from build123d import *

# Parameters (mm, degrees)
SKETCH1_R           = 1.75
SKETCH1_R_2         = 11.5
BOSS_EXTRUDE1_DEPTH = 3.55


with BuildPart() as part:
    # Sketch1 → Boss-Extrude1 (new, symmetric)
    with BuildSketch(Plane.XY):
        Polygon((21.15, -17.614466094), (21.15, 17.614466094), (17.614466094, 21.15), (-17.614466094, 21.15), (-21.15, 17.614466094), (-21.15, -17.614466094), (-17.614466094, -21.15), (17.614466094, -21.15), align=None)
        with Locations((-15.5, 15.5)):
            Circle(SKETCH1_R, mode=Mode.SUBTRACT)
        with Locations((15.5, 15.5)):
            Circle(SKETCH1_R, mode=Mode.SUBTRACT)
        with Locations((15.5, -15.5)):
            Circle(SKETCH1_R, mode=Mode.SUBTRACT)
        with Locations((-15.5, -15.5)):
            Circle(SKETCH1_R, mode=Mode.SUBTRACT)
        Circle(SKETCH1_R_2, mode=Mode.SUBTRACT)
    extrude(amount=BOSS_EXTRUDE1_DEPTH, both=True)


solid = part.part
Design review of the part built by this model. Coordinates are the model's own, in mm. Round coordinates to 2 decimals unless told otherwise and drop trailing zeros. Write each loop counter-clockwise with the first axis right and the second up, starting at its lowest first coordinate (ties: lowest second). Pieces come first, ordered by that corner, then holes. Notation, with made-up numbers: (55.25, 57) - (66.25, 57) arc R7 cw to (66.25, 62) - close; hole circle Ø1 at (-22, -18). An arc over 180 degrees is marked (long way). Use a Markdown table: item, result. Add a question column.
1. We need section C-C (z = -0.5). State the section outline as (x, y) points.
2. Wall thickness on probe 1 along Y at (x, z) = (-15.5, 0); probe 2 along Y at (x, z) = (0, 0.75); probe 3 along Y at (x, z) = (-14, -3): over which ranges is each line inside the solid? List them lowest first.
3. Mouldability with a two-part tool opening along Y and no side actions: class faces 1 (the face through (-1.5, 11.4, 0)), 2 (the face through (-14.6, -14, 0)), 3 (the face through (-21.15, 0, 0)), 4 (the face through (-19.407, -19.357, 0.05)) as +Y half, -Y half, draft (parallel to the pull), parting line (faces both ways), or undercut.
4. We need section B-B (x = 15.5). State the section outline as (y, z) points, then the cut area to 3 significant figures.
5. We need section A-A (y = 0). State the section outline as (x, z) points, then the cut area to 3 significant figures.
Output:
| question | item | result |
|---|---|---|
| 1 | outline | (-21.15, -17.61) - (-17.61, -21.15) - (17.61, -21.15) - (21.15, -17.61) - (21.15, 17.61) - (17.61, 21.15) - (-17.61, 21.15) - (-21.15, 17.61) - close; hole circle Ø3.5 at (-15.5, -15.5); hole circle Ø3.5 at (-15.5, 15.5); hole circle Ø23 at (0, 0); hole circle Ø3.5 at (15.5, -15.5); hole circle Ø3.5 at (15.5, 15.5) |
| 2 | probe 1 | y = -21.15 to -17.25, -13.75 to 13.75, 17.25 to 21.15 |
| 2 | probe 2 | y = -21.15 to -11.5, 11.5 to 21.15 |
| 2 | probe 3 | y = -21.15 to -16.4, -14.6 to 14.6, 16.4 to 21.15 |
| 3 | face 1 | undercut |
| 3 | face 2 | undercut |
| 3 | face 3 | draft |
| 3 | face 4 | -Y half |
| 4 | outline | (-21.15, -3.55) - (-17.25, -3.55) - (-17.25, 3.55) - (-21.15, 3.55) - close; (-13.75, -3.55) - (13.75, -3.55) - (13.75, 3.55) - (-13.75, 3.55) - close; (17.25, -3.55) - (21.15, -3.55) - (21.15, 3.55) - (17.25, 3.55) - close |
| 4 | area | 251 mm2 |
| 5 | outline | (-21.15, -3.55) - (-11.5, -3.55) - (-11.5, 3.55) - (-21.15, 3.55) - close; (11.5, -3.55) - (21.15, -3.55) - (21.15, 3.55) - (11.5, 3.55) - close |
| 5 | area | 137 mm2 |
